Could you check a few things on this model? Use its own coordinates, in mm. Face numbers are marked on the shaded views. Give positions to 0.01 mm unless a question says otherwise; leave off trailing zeros. Loops run counter-clockwise (first coordinate to the right, second up) from the corner with the lowest first, then second, coordinate; pieces in that order, holes last. Notation, with made-up numbers: M 14.25,34 L 29.25,34 A20 cw 29.25,50 Z; hole C 59.5,5 d4. An arc over 180 degrees is marked long. Return JSON: item names as keys, results as strings. Group by question number.
1. If we mould it in two halves opening along X, with no side actions, what happens to the marked faces 1, 2 and 3? For each: +X half, -X half, draft (parallel to the pull), parting line (faces both ways), or undercut.
2. For pin 1 (2 mm diameter, centred on x = -18.5, y = 9, fed in from -Z); pin 2 (1.5 mm diameter, centred on y = 14.5, z = -19.5, fed in from -X); pin 3 (8 mm diameter, centred on y = 12, z = 13, fed in from -X), each with a flat end and sliding along its axis, tell me the tip position at first contact or that it passes through.
3. If we section it at B-B (x = 0): Write out the boundary of the cut face in (y, z) (1 decimal), plus the area to 3 significant figures.
4. If we section it at D-D (y = 13): Write out the boundary of the cut face in (x, z), plus the area to 3 significant figures.
5. Please list where these lines run through material, in increasing order: line 1 (Z direction, x = 0, y = 6); line 2 (Z direction, x = 0, y = 11.5).
6. If we section it at A-A (y = 4.75): Write out the boundary of the cut face in (x, z) (1 decimal).
7. If we section it at C-C (z = 0): Write out the boundary of the cut face in (x, y) (1 decimal), plus the area to 3 significant figures.
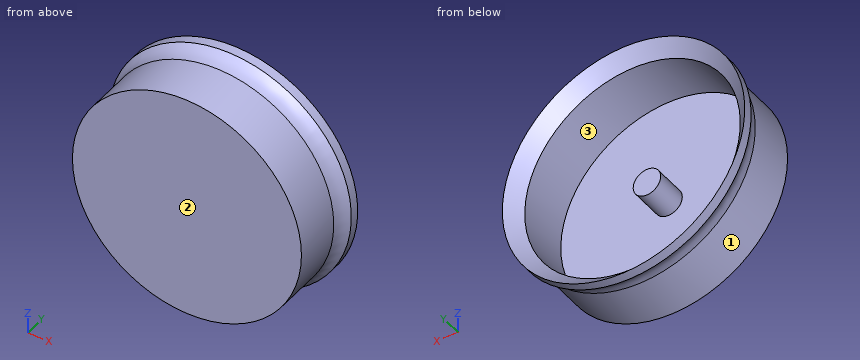
```python
from build123d import *


with BuildPart() as part:
    # Sketch2 → Revolve1 (revolve)
    with BuildSketch(Plane(origin=(0, 0, 0), x_dir=(0, 0, -1), z_dir=(1, 0, 0))):
        with BuildLine():
            Line((0, 0), (0, 9.2075))
            Line((0, 9.2075), (3.2385, 9.2075))
            Line((3.2385, 9.2075), (3.2385, 1.5875))
            Line((3.2385, 1.5875), (25.4, 1.5875))
            Line((25.4, 1.5875), (25.4, 14.2875))
            Line((25.4, 14.2875), (28.575, 17.4625))
            Line((28.575, 17.4625), (28.575, 15.21743597))
            ThreePointArc((28.575, 15.21743597), (27.400077808, 13.459040646), (26.9875, 11.384871939))
            Line((26.9875, 11.384871939), (26.9875, 0))
            Line((26.9875, 0), (0, 0))
        make_face()
    revolve(axis=Axis((0, 0, 0), (0, 1, 0)))


solid = part.part
```
Answer:
{
 "1": {"face 1": "parting line", "face 2": "draft", "face 3": "undercut"},
 "2": {"pin 1": "stops at z = -20.54", "pin 2": "stops at x = -21.15", "pin 3": "stops at x = -26.53"},
 "3": {"outline": "M 0,-27 L 11.4,-27 A5.4 cw 15.2,-28.6 L 17.5,-28.6 L 14.3,-25.4 L 1.6,-25.4 L 1.6,-3.2 L 9.2,-3.2 L 9.2,3.2 L 1.6,3.2 L 1.6,25.4 L 14.3,25.4 L 17.5,28.6 L 15.2,28.6 A5.4 cw 11.4,27 L 0,27 Z", "area": "186 mm²"},
 "4": {"outline": "C 0,0 d54.47; hole C 0,0 d50.8", "area": "303 mm²"},
 "5": {"line 1": "z = -26.99 to -25.4, -3.24 to 3.24, 25.4 to 26.99", "line 2": "z = -26.99 to -25.4, 25.4 to 26.99"},
 "6": {"outline": "C 0,0 d54; C 0,0 d6.5; hole C 0,0 d50.8"},
 "7": {"outline": "M -28.6,15.2 A5.4 cw -27,11.4 L -27,0 L 27,0 L 27,11.4 A5.4 cw 28.6,15.2 L 28.6,17.5 L 25.4,14.3 L 25.4,1.6 L 3.2,1.6 L 3.2,9.2 L -3.2,9.2 L -3.2,1.6 L -25.4,1.6 L -25.4,14.3 L -28.6,17.5 Z", "area": "186 mm²"}
}
